Geometry: final body of the model. Coordinates: model frame, mm. Face numbers are marked on the shaded views. A direction names the side the tool comes from. Give positions to 0.01 mm unless a question says otherwise; leave off trailing zeros. Write each loop counter-clockwise with the first axis right and the second up, starting at its lowest first coordinate (ties: lowest second). Pieces come first, ordered by that corner, then holes. Notation, with made-up numbers: M 29,-15 L 52,-15 A37 ccw 52,21 Z; hole C 60.25,13.25 d7. An arc over 180 degrees is marked long. Use a Markdown table: item, result. Add a question column.
1) Draft query along Z for the marked faces 1, 2 and 3. Return one class per face: +Z half, -Z half, draft (parallel to the pull), parting line (faces both ways), or undercut.
2) Set-up query: the marked faces 4 and 5. Return all of +Z, -Z, +X, -X, +Y, -Y with unobstructed straight access to the full face (end or side cutting, diameter ignored); none if empty.
3) Pin query (flat end, axial travel): pin 1 (6 mm diameter, centred on y = 7, z = 3.5, fed in from +X); pin 2 (3 mm diameter, centred on y = 4.5, z = -3, fed in from -X); pin 3 (5 mm diameter, centred on x = 2.5, y = 0.5, fed in from +Z); pin 4 (3 mm diameter, centred on x = -1.5, z = 0.5, fed in from -Y) (3 decimals). Return the tip coordinate at first contact, or that it passes through.
4) Section B-B on z = -7. Return the cut outline in (x, y) (3 decimals).
5) Line query: line 1 (Z direction, x = 0, y = -0.5); line 2 (Z direction, x = 1.25, y = 0.5); line 3 (Y direction, x = -5.5, z = 0.75) (3 decimals). Output: solid intervals per line, ascending.
6) Section A-A on y = -0.25. Return the cut outline in (x, z) (1 decimal).
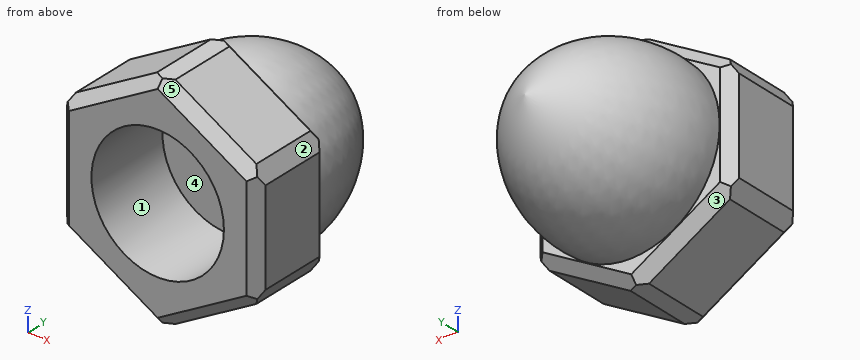
```python
from build123d import *

# Parameters (mm, degrees)
F1_DEPTH = 3.175
F2_R     = 4.7625
F3_DEPTH = 25
F4_SIZE  = 0.762
F5_SIZE  = 0.762
F6_SIZE  = 0.762


with BuildPart() as f1:
    # F0 (on Front) → F1 (new body, symmetric)
    with BuildSketch(Plane.XZ):
        Polygon((-7.14375, 4.1244459855), (-7.14375, -4.1244459855), (0, -8.248891971), (7.14375, -4.1244459855), (7.14375, 4.1244459855), (0, 8.248891971), align=None)
    extrude(amount=F1_DEPTH, both=True)

    # F2 (on face) → F3 (cut)
    with BuildSketch(Plane.XZ.offset(3.175)):
        Circle(F2_R)
    extrude(amount=-F3_DEPTH, mode=Mode.SUBTRACT)

    # F4
    f4_edges = [f1.edges().sort_by_distance(p)[0] for p in [
        (0, 0, 8.248892),
        (7.14375, 0, 4.124446),
        (7.14375, 0, -4.124446),
        (0, 0, -8.248892),
        (-7.14375, 0, -4.124446),
        (-7.14375, 0, 4.124446),
    ]]
    chamfer(f4_edges, length=F4_SIZE)

    # F5 (call 1 of 6: OpenCascade refuses the feature's edges together)
    f5_edges = [f1.edges().sort_by_distance(p)[0] for p in [
        (-3.571875, -3.175, -6.186669),
    ]]
    chamfer(f5_edges, length=F5_SIZE)

    # F5#2 (call 2 of 6)
    f5_2_edges = [f1.edges().sort_by_distance(p)[0] for p in [
        (3.571875, -3.175, -6.186669),
    ]]
    chamfer(f5_2_edges, length=F5_SIZE)

    # F5#3 (call 3 of 6)
    f5_3_edges = [f1.edges().sort_by_distance(p)[0] for p in [
        (7.14375, -3.175, 0),
    ]]
    chamfer(f5_3_edges, length=F5_SIZE)

    # F5#4 (call 4 of 6)
    f5_4_edges = [f1.edges().sort_by_distance(p)[0] for p in [
        (3.571875, -3.175, 6.186669),
    ]]
    chamfer(f5_4_edges, length=F5_SIZE)

    # F5#5 (call 5 of 6)
    f5_5_edges = [f1.edges().sort_by_distance(p)[0] for p in [
        (-3.571875, -3.175, 6.186669),
    ]]
    chamfer(f5_5_edges, length=F5_SIZE)

    # F5#6 (call 6 of 6)
    f5_6_edges = [f1.edges().sort_by_distance(p)[0] for p in [
        (-7.14375, -3.175, 0),
    ]]
    chamfer(f5_6_edges, length=F5_SIZE)

    # F6 (call 1 of 6: OpenCascade refuses the feature's edges together)
    f6_edges = [f1.edges().sort_by_distance(p)[0] for p in [
        (-3.571875, 3.175, -6.186669),
    ]]
    chamfer(f6_edges, length=F6_SIZE)

    # F6#2 (call 2 of 6)
    f6_2_edges = [f1.edges().sort_by_distance(p)[0] for p in [
        (3.571875, 3.175, -6.186669),
    ]]
    chamfer(f6_2_edges, length=F6_SIZE)

    # F6#3 (call 3 of 6)
    f6_3_edges = [f1.edges().sort_by_distance(p)[0] for p in [
        (7.14375, 3.175, 0),
    ]]
    chamfer(f6_3_edges, length=F6_SIZE)

    # F6#4 (call 4 of 6)
    f6_4_edges = [f1.edges().sort_by_distance(p)[0] for p in [
        (3.571875, 3.175, 6.186669),
    ]]
    chamfer(f6_4_edges, length=F6_SIZE)

    # F6#5 (call 5 of 6)
    f6_5_edges = [f1.edges().sort_by_distance(p)[0] for p in [
        (-3.571875, 3.175, 6.186669),
    ]]
    chamfer(f6_5_edges, length=F6_SIZE)

    # F6#6 (call 6 of 6)
    f6_6_edges = [f1.edges().sort_by_distance(p)[0] for p in [
        (-7.14375, 3.175, 0),
    ]]
    chamfer(f6_6_edges, length=F6_SIZE)

    # F7 (on Top) → F8 (revolve)
    with BuildSketch(Plane.XY):
        with BuildLine():
            Line((0, 12.7), (0, 3.175))
            Line((0, 3.175), (6.35, 3.175))
            ThreePointArc((6.35, 3.175), (4.8788606959, 9.0734071306), (0, 12.7))
        make_face()
    revolve(axis=Axis((0, 7.9375, 0), (0, 1, 0)))


solid = f1.part
```
Found:
| question | item | result |
|---|---|---|
| 1 | face 1 | undercut |
| 1 | face 2 | +Z half |
| 1 | face 3 | -Z half |
| 2 | face 4 | -Y |
| 2 | face 5 | +Z, +X, -Y |
| 3 | pin 1 | x = 6.23 |
| 3 | pin 2 | x = -6.56 |
| 3 | pin 3 | z = 7.87 |
| 3 | pin 4 | y = 3.175 |
| 4 | outline | M -2.163,-2.413 L -0.639,-3.175 L 0.639,-3.175 L 2.163,-2.413 L 2.163,2.413 L 0.639,3.175 L -0.639,3.175 L -2.163,2.413 Z |
| 5 | line 1 | -7.87 to -4.76, 4.76 to 7.87 |
| 5 | line 2 | -7.53 to -4.6, 4.6 to 7.53 |
| 5 | line 3 | -3.175 to 7.877 |
| 6 | outline | M -7.1,-3.4 L -6.5,-4.5 L -0.7,-7.9 L 0.7,-7.9 L 6.5,-4.5 L 7.1,-3.4 L 7.1,3.4 L 6.5,4.5 L 0.7,7.9 L -0.7,7.9 L -6.5,4.5 L -7.1,3.4 Z; hole C 0,0 d9.5 |
